The figure shows three views and two pictorial views of one solid part (mm, origin at its lowest corner). Answer the questions. A direction names the side the tool comes from. Coordinates: 2 decimals unless noted, no trailing zeros. Write each loop counter-clockwise with the first axis right and the second up, starting at its lowest first coordinate (ties: lowest second). Pieces come first, ordered by that corner, then holes. Notation, with made-up numbers: (21.5, 81.5) - (31.5, 81.5) arc R16 ccw to (31.5, 99.5) - close; hole circle Ø5 at (37.25, 27.25). An arc over 180 degrees is marked (long way). Use a Markdown table: item, result. Add a question column.
(1) Given pin 1 Ø9.5 at (x, y) = (27.5, 14) entering from -Z; pin 2 Ø1.5 at (x, z) = (33, 6.5) entering from -Y; pin 3 Ø15 at (y, z) = (33, 47) entering from -X; pin 4 Ø2 at (x, y) = (13, 16.5) entering from +Z, each flat-ended and moving along its own axis, determine where each tip first touches the part or whether it passes through.
(2) The part is cut by section B-B, the plane z = 23. Give the vertices of the cut face in (x, y), then the cut area to 3 significant figures.
(3) The part is cut by section A-A, the plane x = 35. Give the vertices of the cut face in (y, z).
(4) The part is cut by section D-D, the plane x = 7. Give the vertices of the cut face in (y, z).
(5) The part is cut by section C-C, the plane y = 30. Give the vertices of the cut face in (x, z).
(6) A tool of negligible diameter and unlimited length cuts with its end or side. For the marked faces 1, 2, 3 and 4, from which of +Z, -Z, +X, -X, +Y, -Y can it reach the whole face along a straight path? Write none if from no direction.
(7) Find the intervals of material crossed by line 1 (X direction, y = 17, z = 34); line 2 (Z direction, x = 8.5, y = 29.5), in increasing order. Write a range as from..to.
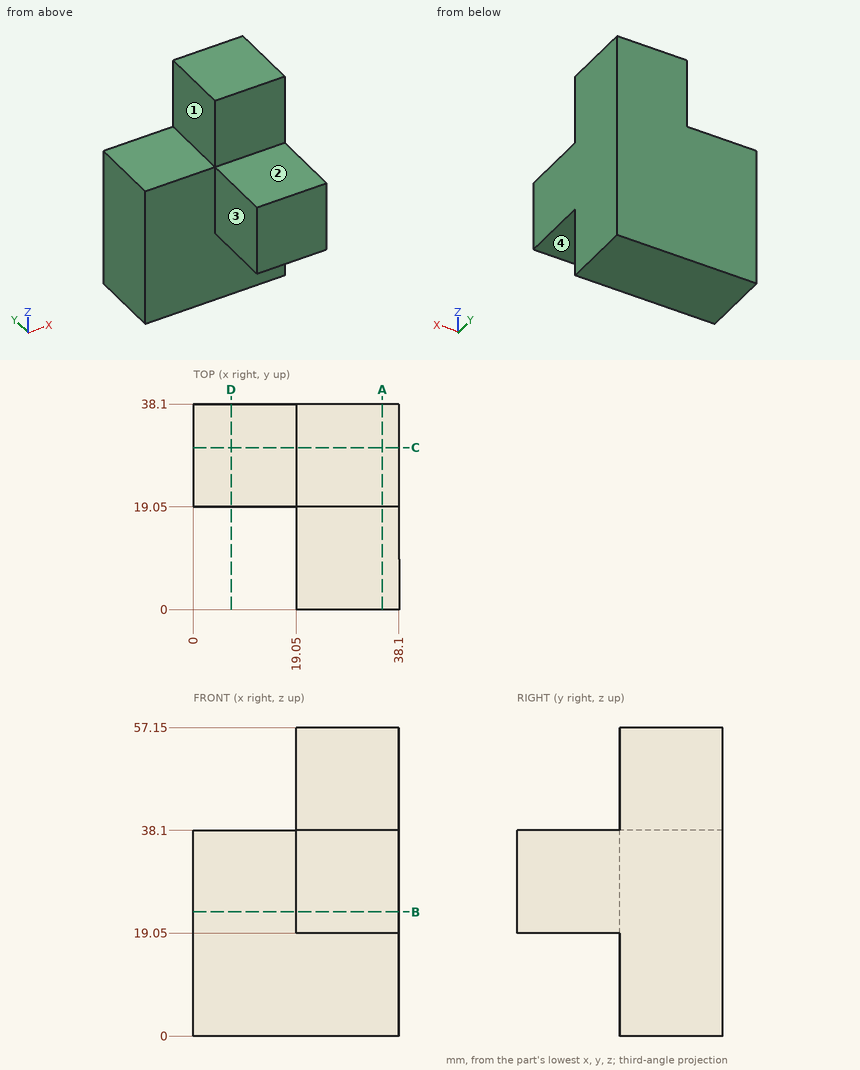
Model answer:
| question | item | result |
|---|---|---|
| 1 | pin 1 | z = 19.05 |
| 1 | pin 2 | y = 19.05 |
| 1 | pin 3 | x = 19.05 |
| 1 | pin 4 | through |
| 2 | outline | (0, 19.05) - (19.05, 19.05) - (19.05, 0) - (38.1, 0) - (38.1, 38.1) - (0, 38.1) - close |
| 2 | area | 1,090 mm^2 |
| 3 | outline | (0, 19.05) - (19.05, 19.05) - (19.05, 0) - (38.1, 0) - (38.1, 57.15) - (19.05, 57.15) - (19.05, 38.1) - (0, 38.1) - close |
| 4 | outline | (19.05, 0) - (38.1, 0) - (38.1, 38.1) - (19.05, 38.1) - close |
| 5 | outline | (0, 0) - (38.1, 0) - (38.1, 57.15) - (19.05, 57.15) - (19.05, 38.1) - (0, 38.1) - close |
| 6 | face 1 | +Z, -X, +Y, -Y |
| 6 | face 2 | +Z, +X, -X, -Y |
| 6 | face 3 | +Z, -Z, -X, -Y |
| 6 | face 4 | -Z, +X, -X, -Y |
| 7 | line 1 | 19.05..38.1 |
| 7 | line 2 | 0..38.1 |
